Build history of the part. All positions in model axes, mm. Face numbers are marked on the shaded views. A direction names the side the tool comes from. Round coordinates to 2 decimals unless told otherwise and drop trailing zeros. Order: outer loops, then holes, each group sorted by start corner. A loop starts at its lowest first (then second) coordinate and runs counter-clockwise, first axis right, second up. Notation, with made-up numbers: (23.25, 73.5) - (82.25, 73.5) arc R17 cw to (82.25, 84.5) - close; hole circle Ø11 at (9, 12). An arc over 180 degrees is marked (long way). One line per question, with ' | ' between items. Start each with the question number.
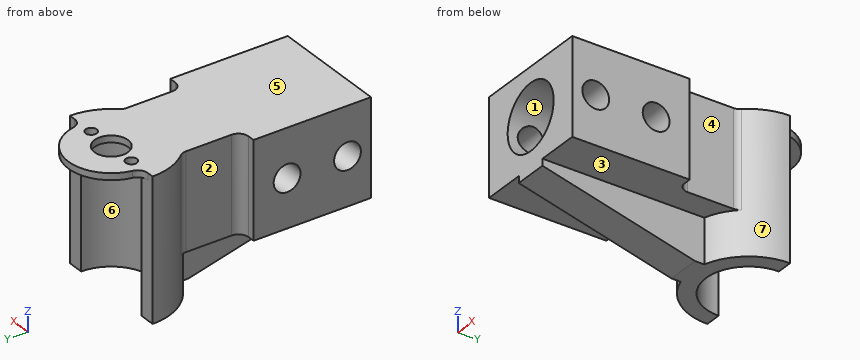
from build123d import *

# Parameters (mm, degrees)
SKETCH2_R               = 12.75
SKETCH2_R_2             = 5
SKETCH2_R_3             = 1.675
BOSS_EXTRUDE3_DEPTH     = 2
BOSS_EXTRUDE4_START     = -40
BOSS_EXTRUDE4_DEPTH     = 42
BOSS_EXTRUDE6_START     = -30
SKETCH7_W               = 35.2
SKETCH7_H               = 28.7
SKETCH7_R               = 9.725
BOSS_EXTRUDE6_DEPTH     = 35
BOSS_EXTRUDE7_START     = -26.7
BOSS_EXTRUDE7_DEPTH     = 26.7
CUT_EXTRUDE1_DEPTH      = 79.324708745
CUT_EXTRUDE1_DEPTH_BACK = 79.324708745
SKETCH6_R               = 4
RIB3_START              = -5
RIB3_DEPTH              = 10
FILLET2_R               = 3


with BuildPart() as part:
    # Sketch2 → Boss-Extrude3 (new body)
    # profile 1 of 2: a face of its own
    with BuildSketch(Plane.XY):
        Circle(SKETCH2_R)
        Circle(SKETCH2_R_2, mode=Mode.SUBTRACT)
        with Locations((8.5, 0)):
            Circle(SKETCH2_R_3, mode=Mode.SUBTRACT)
        with Locations((-8.5, 0)):
            Circle(SKETCH2_R_3, mode=Mode.SUBTRACT)
    # profile 2 of 2: a face of its own
    with BuildSketch(Plane.XY):
        with BuildLine():
            Line((12.5, -30), (12.5, -2.512468905))
            ThreePointArc((12.5, -2.512468905), (0, -12.75), (-12.5, -2.512468905))
            Line((-12.5, -2.512468905), (-12.5, -30))
            Line((-12.5, -30), (12.5, -30))
        make_face()
    extrude(amount=BOSS_EXTRUDE3_DEPTH)

    # Sketch3 → Boss-Extrude4 (add)
    with BuildSketch(Plane.XY.offset(BOSS_EXTRUDE4_START)):
        with BuildLine():
            Line((17.5, 0), (12.75, 0))
            ThreePointArc((12.75, 0), (0, -12.75), (-12.75, 0))
            Line((-12.75, 0), (-17.5, 0))
            ThreePointArc((-17.5, 0), (0, -17.5), (17.5, 0))
        make_face()
    extrude(amount=BOSS_EXTRUDE4_DEPTH)

    # Sketch7 → Boss-Extrude6 (add)
    with BuildSketch(Plane(origin=(0, 0, 0), x_dir=(1, 0, 0), z_dir=(0, 1, 0)).offset(BOSS_EXTRUDE6_START)):
        with Locations((0, 12.35)):
            Rectangle(SKETCH7_W, SKETCH7_H)
        with Locations(Location((0, 12.35, 0), (0, 0, 180))):
            Circle(SKETCH7_R, mode=Mode.SUBTRACT)
    extrude(amount=-BOSS_EXTRUDE6_DEPTH)

    # Sketch2<8> → Boss-Extrude7 (add)
    with BuildSketch(Plane.XY.offset(BOSS_EXTRUDE7_START)):
        with BuildLine():
            Line((12.5, -30), (12.5, -2.512468905))
            ThreePointArc((12.5, -2.512468905), (0, -12.75), (-12.5, -2.512468905))
            Line((-12.5, -2.512468905), (-12.5, -30))
            Line((-12.5, -30), (12.5, -30))
        make_face()
    extrude(amount=BOSS_EXTRUDE7_DEPTH)

    # Sketch6 → Cut-Extrude1 (cut, two sides: drawn at the far end of the back side and taken through both)
    with BuildSketch(Plane(origin=(0, 0, 0), x_dir=(0, 0, -1), z_dir=(1, 0, 0)).offset(-CUT_EXTRUDE1_DEPTH_BACK)):
        with Locations((12.35, -40)):
            Circle(SKETCH6_R)
        with Locations((12.35, -58)):
            Circle(SKETCH6_R)
    extrude(amount=CUT_EXTRUDE1_DEPTH + CUT_EXTRUDE1_DEPTH_BACK, mode=Mode.SUBTRACT)

    # Rib3: read off the stored shape, not the designer's step
    # Rib3 outline → Rib3 (add)
    with BuildSketch(Plane(origin=(0, -60, 0), x_dir=(0, -1, 0), z_dir=(-1, 0, 0)).offset(RIB3_START)):
        Polygon((5, -28.7), (5, -26.7), (-43.229490169, -26.7), (-43.229490169, -40), (-40.5, -40), align=None)
    extrude(amount=RIB3_DEPTH)

    # Fillet2
    fillet2_edges = [part.edges().sort_by_distance(p)[0] for p in [
        (12.5, -30, -12.35),
        (-12.5, -30, -12.35),
        (-12.75, 0, 1),
        (12.5, -12.247448714, -12.35),
        (12.75, 0, 1),
        (-12.5, -12.247448714, -12.35),
    ]]
    fillet(fillet2_edges, radius=FILLET2_R)


solid = part.part
Item 1: 3-axis set-ups, long thin cutter, end or side, ignore diameter. For the marked faces 1, 2, 3 and 4: which of +Z, -Z, +X, -X, +Y, -Y reach the whole face in a straight line?
Item 2: Pull direction X, two halves, no side cores. Call the marked faces 5, 6 and 7: released by +X, released by -X, zero draft, split by the parting line, or undercut.
Item 3: Pin check, flat tips, straight feed: pin 1 (17.5 mm diameter, centred on x = 0, z = -12.35, fed in from -Y); pin 2 (1.5 mm diameter, centred on x = 2.5, z = -28.5, fed in from +Y); pin 3 (2.5 mm diameter, centred on x = -17, z = -14.5, fed in from +Y); pin 4 (3 mm diameter, centred on x = 8.5, y = 0, fed in from -Z). Stop position of each tip, or through.
Item 4: Slice it at B-B (z = -12.35). Count the separate pieces of the cut face and the enclosed holes in it, plus the area to 3 significant figures.
Item 5: Wall check: line 1 along X through (y, z) = (-49, -12); line 2 along Z through (x, y) = (-11, -58); line 3 along Y through (x, z) = (13.75, -12.35). Give the ranges that are in metal, low to high. Write a range as [from, to].
Item 6: Slice it at D-D (z = -6). Write the cut outline in (x, y), plus the area to 3 significant figures.
Item 7: Slice it at A-A (y = -58). Write the cut outline in (x, z) (3 decimals), plus the area to 3 significant figures.
Item 8: Slice it at C-C (x = 8). Write the cut outline in (y, z).
A:
1) face 1: -Y | face 2: +Z, -Z, -X | face 3: -Z, +X, -Y | face 4: +Z, -Z, +X
2) face 5: zero draft | face 6: undercut | face 7: released by +X
3) pin 1: y = -30 | pin 2: y = -12.33 | pin 3: y = 0 | pin 4: through
4) separate pieces: 5 | enclosed holes: 0 | area: 882 mm^2
5) line 1: [-17.6, -9.72], [9.72, 17.6] | line 2: [-26.7, -16.35], [-8.35, 2] | line 3: [-65, -62], [-54, -44], [-36, -29.44], [-10.83, 0]
6) outline: (-17.6, -65) - (-7.37, -65) - (-7.37, -30) - (7.37, -30) - (7.37, -65) - (17.6, -65) - (17.6, -30) - (15.5, -30) arc R3 cw to (12.5, -27) - (12.5, -13.42) arc R3 cw to (13.23, -11.45) arc R17.5 ccw to (17.5, 0) - (12.75, 0) arc R12.75 cw to (-12.75, 0) - (-17.5, 0) arc R17.5 ccw to (-13.23, -11.45) arc R3 cw to (-12.5, -13.42) - (-12.5, -27) arc R3 cw to (-15.5, -30) - (-17.6, -30) - close | area: 1,300 mm^2
7) outline: (-17.6, -26.7) - (-5, -26.7) - (-5, -30.438) - (5, -30.438) - (5, -26.7) - (17.6, -26.7) - (17.6, -16.35) - (8.864, -16.35) arc R9.725 cw to (-8.864, -16.35) - (-17.6, -16.35) - close; (-17.6, -8.35) - (-8.864, -8.35) arc R9.725 cw to (8.864, -8.35) - (17.6, -8.35) - (17.6, 2) - (-17.6, 2) - close | area: 620 mm^2
8) outline: (-65, -26.7) - (-15.56, -26.7) - (-15.56, -40) - (-9.93, -40) - (-9.93, 0) - (-1.6, 0) - (-1.6, 2) - (-65, 2) - (-65, -6.82) - (-30, -6.82) - (-30, -17.88) - (-65, -17.88) - close; (1.6, 0) - (9.93, 0) - (9.93, 2) - (1.6, 2) - close
